CAD build for the part. Positions are in the model's coordinates, mm. A direction names the side the tool comes from. Round coordinates to 2 decimals unless told otherwise and drop trailing zeros. Loops run counter-clockwise (first coordinate to the right, second up) from the corner with the lowest first, then second, coordinate; pieces in that order, holes last. Notation, with made-up numbers: M 89,0 L 122,0 A11 ccw 122,6 Z; hole C 58,-3 d9. An arc over 180 degrees is marked long. Use one line per item in the form item = value.
from build123d import *

# Parameters (mm, degrees)
BOSS_EXTRUDE1_DEPTH   = 20
SKETCH2_R             = 2
CUT_EXTRUDE1_DEPTH    = 20
SKETCH3_R             = 2
BOSS_EXTRUDE3_DEPTH   = 20
BOSS_EXTRUDE3_2_DEPTH = 20
CUT_EXTRUDE3_START    = -20
SKETCH4_R             = 2
CUT_EXTRUDE3_DEPTH    = 20
CUT_EXTRUDE4_START    = -29
SKETCH4_2_R           = 2
CUT_EXTRUDE4_DEPTH    = 29
CUT_EXTRUDE6_START    = -20
CUT_EXTRUDE6_DEPTH    = 20
BOSS_EXTRUDE4_START   = -1
BOSS_EXTRUDE4_DEPTH   = 1
BOSS_EXTRUDE5_START   = -1
SKETCH7_R             = 2
BOSS_EXTRUDE5_DEPTH   = 1
SKETCH8_R             = 2
CUT_EXTRUDE7_DEPTH    = 1


with BuildPart() as part:
    # Sketch1 → Boss-Extrude1 (new body)
    with BuildSketch(Plane.XY):
        with BuildLine():
            Line((12.5, 0), (30, 0))
            Line((30, 0), (30, -1))
            Line((30, -1), (13.462912018, -1))
            ThreePointArc((13.462912018, -1), (0, -13.5), (-13.462912018, -1))
            Line((-13.462912018, -1), (-30, -1))
            Line((-30, -1), (-30, 0))
            Line((-30, 0), (-12.5, 0))
            ThreePointArc((-12.5, 0), (0, -12.5), (12.5, 0))
        make_face()
    extrude(amount=BOSS_EXTRUDE1_DEPTH)

    # Sketch2 → Cut-Extrude1 (cut)
    with BuildSketch(Plane(origin=(0, 0, 0), x_dir=(1, 0, 0), z_dir=(0, 1, 0))):
        with Locations(Location((20, -10, 0), (0, 0, 270))):
            Circle(SKETCH2_R)
        with BuildLine():
            ThreePointArc((30, -10), (28.962912018, -15.385164807), (26, -20))
            Line((26, -20), (30, -20))
            Line((30, -20), (30, -10))
        make_face()
        with BuildLine():
            Line((30, 0), (26, 0))
            ThreePointArc((26, 0), (28.962912018, -4.614835193), (30, -10))
            Line((30, -10), (30, 0))
        make_face()
        with BuildLine():
            Line((-30, 0), (-30, -9.99999978))
            ThreePointArc((-30, -9.99999978), (-28.962911977, -4.614835091), (-26, 0))
            Line((-26, 0), (-30, 0))
        make_face()
        with BuildLine():
            Line((-30, -20), (-26, -20))
            ThreePointArc((-26, -20), (-28.962912059, -15.385164705), (-30, -9.99999978))
            Line((-30, -9.99999978), (-30, -20))
        make_face()
        with Locations(Location((-26, -10, 0), (0, 0, 270))):
            Circle(SKETCH2_R)
    extrude(amount=-CUT_EXTRUDE1_DEPTH, mode=Mode.SUBTRACT)

    # Sketch4_2 → Cut-Extrude4 (cut)
    with BuildSketch(Plane.XZ.offset(21).offset(CUT_EXTRUDE4_START)):
        with Locations(Location((20, 10, 0), (0, 0, 90))):
            Circle(SKETCH4_2_R)
        with Locations((-24, 10)):
            Circle(SKETCH4_2_R)
    extrude(amount=CUT_EXTRUDE4_DEPTH, mode=Mode.SUBTRACT)

    # Sketch6 → Boss-Extrude4 (add)
    with BuildSketch(Plane.XZ.offset(1).offset(BOSS_EXTRUDE4_START)):
        with BuildLine():
            ThreePointArc((-25, 11.732050808), (-26, 10), (-25, 8.267949192))
            ThreePointArc((-25, 8.267949192), (-28, 10), (-25, 11.732050808))
        make_face()
    extrude(amount=BOSS_EXTRUDE4_DEPTH)

    # Sketch7 → Boss-Extrude5 (add)
    with BuildSketch(Plane.XZ.offset(1).offset(BOSS_EXTRUDE5_START)):
        with Locations((20, 10)):
            Circle(SKETCH7_R)
    extrude(amount=BOSS_EXTRUDE5_DEPTH)

    # Sketch8 → Cut-Extrude7 (cut)
    with BuildSketch(Plane.XZ.offset(1)):
        with Locations(Location((24, 10, 0), (0, 0, 270))):
            Circle(SKETCH8_R)
    extrude(amount=-CUT_EXTRUDE7_DEPTH, mode=Mode.SUBTRACT)


with BuildPart() as body_2:
    # Sketch3 → Boss-Extrude3 (new body)
    with BuildSketch(Plane.XZ.offset(1)):
        with Locations(Location((20, 10, 0), (0, 0, 90))):
            Circle(SKETCH3_R)
    extrude(amount=BOSS_EXTRUDE3_DEPTH)

    # Sketch4 → Cut-Extrude3 (cut)
    with BuildSketch(Plane.XZ.offset(21).offset(CUT_EXTRUDE3_START)):
        with Locations(Location((20, 10, 0), (0, 0, 90))):
            Circle(SKETCH4_R)
        with Locations((-24, 10)):
            Circle(SKETCH4_R)
    extrude(amount=CUT_EXTRUDE3_DEPTH, mode=Mode.SUBTRACT)


with BuildPart() as body_3:
    # Sketch3 → Boss-Extrude3 2 (new body)
    with BuildSketch(Plane.XZ.offset(1)):
        with BuildLine():
            ThreePointArc((-25, 8.267949192), (-26, 10), (-25, 11.732050808))
            ThreePointArc((-25, 11.732050808), (-28, 10), (-25, 8.267949192))
        make_face()
    extrude(amount=BOSS_EXTRUDE3_2_DEPTH)

    # Sketch5 → Cut-Extrude6 (cut)
    with BuildSketch(Plane.XZ.offset(21).offset(CUT_EXTRUDE6_START)):
        with BuildLine():
            ThreePointArc((-25, 11.732050808), (-28, 10), (-25, 8.267949192))
            ThreePointArc((-25, 8.267949192), (-26, 10), (-25, 11.732050808))
        make_face()
    extrude(amount=CUT_EXTRUDE6_DEPTH, mode=Mode.SUBTRACT)


solid = part.part
1. Tool access for faces 5 (the face through (0, -13, 20)), 6 (the face through (21.8, -1, 9.9)): list every direction of +Z, -Z, +X, -X, +Y, -Y with a clear straight run to the whole face (end or side of a thin tool).
Completed:
face_5 = +Z, +X, -X, +Y, -Y
face_6 = +Z, -Z, +X, -Y
2. Cut at A-A on y = -2.5. Write the cut outline in (x, z), and give its area (3 significant figures).
Completed:
outline = M -13.27,0 L -12.25,0 L -12.25,20 L -13.27,20 Z; M 12.25,0 L 13.27,0 L 13.27,20 L 12.25,20 Z
area = 40.8 mm2
3. Drop flat-ended pins along their axis: P1, Ø12, axis at x = 10, z = 14, coming from the -Y side; P2, Ø3, axis at y = -2, z = 12, coming from the +X side; P3, Ø5, axis at x = 20.5, z = 6.5, coming from the -Y side. Give the stop position or say it passes through.
Completed:
P1 = -12.89
P2 = 29.97
P3 = -1
4. Cut at D-D on x = -17. Write the cut outline in (y, z), and give its area (3 significant figures).
Completed:
outline = M -1,0 L 0,0 L 0,20 L -1,20 Z
area = 20.0 mm2
5. Cut at B-B on x = 24. Write the cut outline in (y, z).
Completed:
outline = M -1,0 L 0,0 L 0,8 L -1,8 Z; M -1,12 L 0,12 L 0,20 L -1,20 Z
6. Pull direction X, two halves, no side cores. Call faces 1 (the face through (22.8, -0.5, 11.6)), 2 (the face through (0.283, -13.497, 9.86)), 3 (the face through (-0.275, -12.497, 9.86)), 4 (the face through (-21.6, -1, 10.1)): +X half, -X half, draft (parallel to the pull), parting line (faces both ways), or undercut.
Completed:
face_1 = undercut
face_2 = parting line
face_3 = undercut
face_4 = draft
7. Probe line 1 along X through (y, z) = (-0.35, 10); line 2 along Z through (x, y) = (-24, -0.45); line 3 along Y through (x, z) = (-26, 4.75). List the from-to ranges inside material, lowest first. Write a range as from..to.
Completed:
line_1 = -30..-26, -22..-12.5, 12.5..22, 26..30
line_2 = 0..8, 12..20
line_3 = -1..0
8. Cut at C-C on z = 13. Write the cut outline in (x, y), and give its area (3 significant figures).
Completed:
outline = M -29.69,-1 L -13.46,-1 A13.5 ccw 13.46,-1 L 29.69,-1 L 29.69,0 L 12.5,0 A12.5 cw -12.5,0 L -29.69,0 Z
area = 73.2 mm2
